```python
from build123d import *

# Parameters (mm, degrees)
F0_W     = 4
F0_H     = 13
F1_DEPTH = 1.6
F2_R     = 15
F3_R     = 5
F4_R     = 1


# Not quite as in the source:
# - a feature names something its author has since deleted; it is built from what else it names


with BuildPart() as f1:
    # F0 (on Front) → F1 (new body)
    with BuildSketch(Plane.XZ):
        Polygon((-19.25, 42), (-23.25, 42), (-23.25, 0), (-20.75, -4.3301270189), (-20.75, -44.8660254038), (20.75, -44.8660254038), (20.75, -4.3301270189), (23.25, 0), (23.25, 42), (19.25, 42), (19.25, 0), (-19.25, 0), align=None)
        with Locations((-11.25, -11.6689147807)):
            Rectangle(F0_W, F0_H, mode=Mode.SUBTRACT)
        with Locations((0, -35.3660254038)):
            Rectangle(F0_W, F0_H, mode=Mode.SUBTRACT)
        with Locations((11.25, -11.6689147807)):
            Rectangle(F0_W, F0_H, mode=Mode.SUBTRACT)
    extrude(amount=F1_DEPTH)

    # F2
    f2_edges = [f1.edges().sort_by_distance(p)[0] for p in [
        (-19.25, -0.8, 0),
        (19.25, -0.8, 0),
        (23.25, -0.8, 0),
        (-23.25, -0.8, 0),
    ]]
    fillet(f2_edges, radius=F2_R)

    # F3
    f3_edges = [f1.edges().sort_by_distance(p)[0] for p in [
        (-20.75, -0.8, -4.330127),
        (20.75, -0.8, -4.330127),
    ]]
    fillet(f3_edges, radius=F3_R)

    # F4
    f4_edges = [f1.edges().sort_by_distance(p)[0] for p in [
        (-13.25, -0.8, -5.168915),
        (-13.25, -0.8, -18.168915),
        (-9.25, -0.8, -5.168915),
        (-9.25, -0.8, -18.168915),
        (13.25, -0.8, -18.168915),
        (13.25, -0.8, -5.168915),
        (9.25, -0.8, -5.168915),
        (9.25, -0.8, -18.168915),
        (-2, -0.8, -41.866025),
        (-2, -0.8, -28.866025),
        (2, -0.8, -28.866025),
        (2, -0.8, -41.866025),
        (20.75, -0.8, -44.866025),
        (-20.75, -0.8, -44.866025),
        (-19.25, -0.8, 42),
        (-23.25, -0.8, 42),
        (19.25, -0.8, 42),
        (23.25, -0.8, 42),
    ]]
    fillet(f4_edges, radius=F4_R)


solid = f1.part
```
Part model, mm, in its own coordinate system. A direction names the side the tool comes from. Give positions to 0.01 mm unless a question says otherwise; leave off trailing zeros. Order: outer loops, then holes, each group sorted by start corner. A loop starts at its lowest first (then second) coordinate and runs counter-clockwise, first axis right, second up. Notation, with made-up numbers: (10.5, 80) - (18.5, 80) arc R22 cw to (18.5, 109) - close; hole circle Ø9 at (-30.5, 40). An arc over 180 degrees is marked (long way). Use one line per item in the form item = value.
Item 1: Pin check, flat tips, straight feed: pin 1 Ø0.5 at (y, z) = (-0.5, -37.5) entering from +X; pin 2 Ø0.8 at (x, y) = (-11, -0.5) entering from +Z; pin 3 Ø0.5 at (y, z) = (-0.5, -10.5) entering from -X. Stop position of each tip, or through.
Solution:
pin_1 = 20.75
pin_2 = 1.81
pin_3 = -20.75
Item 2: Slice it at A-A on z = 23.5. Give the cut face in (x, y), and give its area (3 significant figures).
Solution:
outline = (-23.25, -1.6) - (-19.25, -1.6) - (-19.25, 0) - (-23.25, 0) - close; (19.25, -1.6) - (23.25, -1.6) - (23.25, 0) - (19.25, 0) - close
area = 12.8 mm2
Item 3: Slice it at B-B on z = -10.5. Give the cut face in (x, y).
Solution:
outline = (-20.75, -1.6) - (-13.25, -1.6) - (-13.25, 0) - (-20.75, 0) - close; (-9.25, -1.6) - (9.25, -1.6) - (9.25, 0) - (-9.25, 0) - close; (13.25, -1.6) - (20.75, -1.6) - (20.75, 0) - (13.25, 0) - close
Item 4: Slice it at C-C on x = -3. Give the cut face in (y, z).
Solution:
outline = (-1.6, -44.87) - (0, -44.87) - (0, 0) - (-1.6, 0) - close
Item 5: Which spindle directions (+Z, -Z, +X, -X, +Y, -Y) get a long thin tool onto all of the face, cutting with end or side? Do faces 4 (the face through (20.75, -1, -25)), 5 (the face through (0, -1, 0)), 6 (the face through (-20.75, -1, -24)), 7 (the face through (-11, -1, -18.169)). Say none if no direction does.
Solution:
face_4 = -Z, +X, +Y, -Y
face_5 = +Z, +Y, -Y
face_6 = -Z, -X, +Y, -Y
face_7 = +Y, -Y
Item 6: Slice it at D-D on y = -0.7. Count the separate pieces of the cut face and the enclosed holes in it, and give its area (3 significant figures).
Solution:
separate_pieces = 1
enclosed_holes = 3
area = 2,150 mm2
Item 7: Two-plate mould, pull along X, no slides. Class faces 1 (the face through (-21, -1, 42)), 2 (the face through (-2, -1, -35)), 3 (the face through (-22.787, -0.811, 0.321)): released by +X, released by -X, zero draft, split by the parting line, or undercut.
Solution:
face_1 = zero draft
face_2 = undercut
face_3 = released by -X
Item 8: Probe probe 1 along X at (y, z) = (-0.1, -13.5); probe 2 along Z at (x, y) = (0, -0.4); probe 3 along X at (y, z) = (-0.1, 24.5). List the from-to ranges inside material, lowest first. Write a range as from..to.
Solution:
probe_1 = -20.75..-13.25, -9.25..9.25, 13.25..20.75
probe_2 = -44.87..-41.87, -28.87..0
probe_3 = -23.25..-19.25, 19.25..23.25
